Autodesk Inventor part; units mm, degrees
ref_plane "Work Plane1" through (-155.5267, -73.0733, 0) normal (-1, 0, 0) x (0, 0, 1)
ref_plane "YZ Plane" through (0, 0, 0) normal (1, 0, 0) x (0, 1, 0)
ref_plane "XZ Plane" through (0, 0, 0) normal (0, 1, 0) x (-1, 0, 0)
sketch "Sketch1" plane through (0, 0, 0) normal (0, 0, 1) x (1, 0, 0)
  line L0 (0, 0) -> (-28.5267, 28.5267) construction
  line L1 (-28.5267, 28.5267) -> (-79.3267, 28.5267)
  line L2 (-79.3267, -73.0733) -> (-28.5267, -123.8733)
  line L3 (-28.5267, -123.8733) -> (-28.5267, -149.2733)
  line L4 (-28.5267, -149.2733) -> (-104.7267, -73.0733)
  line L5 (-104.7267, -73.0733) -> (-104.7267, 79.3267)
  line L6 (-79.3267, -73.0733) -> (-79.3267, 28.5267)
  line L7 (-28.5267, 28.5267) -> (-28.5267, 79.3267)
  line L8 (-28.5267, 79.3267) -> (-104.7267, 79.3267)
  point P0 (-28.5267, 153.9136)
  dimension "d11" = 101.6
  dimension "d12" = 50.8
  dimension "d13" = 25.4
  dimension "d17" = 28.5267
  dimension "d18" = 50.8
  dimension "d23" = 135
  dimension "d24" = 17.9605
  dimension "d25" = 50.8
  dimension "d26" = 152.4
extrude "Extrusion1" add sketch "Sketch1" along normal blind 76.2
ref_plane "Work Plane1" through (-155.5267, -73.0733, 0) normal (-1, 0, 0) x (0, 0, 1)
sketch "Sketch2" plane through (-155.5267, -73.0733, 0) normal (-1, 0, 0) x (0, 0, 1)
  line L0 (0, -76.2) -> (76.2, -76.2)
  line L1 (76.2, -76.2) -> (50.8, -76.2)
  line L2 (76.2, 0) -> (76.2, 101.6)
  line L3 (50.8, -76.2) -> (76.2, 0)
  line L4 (76.2, 0) -> (76.2, -76.2)
  line L5 (0, 0) -> (0, -76.2)
  line L6 (0, -76.2) -> (25.4, -76.2)
  line L7 (25.4, -76.2) -> (0, 0)
  line L8 (0, 0) -> (0, -76.2)
  point P0 (0, 73.0733)
  dimension "d28" = 25.4
  dimension "d29" = 25.4
extrude "Extrusion2" cut sketch "Sketch2" against normal blind 177.8
sketch "Sketch3" plane through (-104.7267, 79.3267, 0) normal (0, 1, 0) x (1, 0, 0)
  circle A0 centre (38.1, -38.1) radius 8.7376
  line L0 (76.2, 0) -> (0, 0)
  line L1 (76.2, 0) -> (76.2, -76.2)
  point P0 (104.7267, 0)
  dimension "d32" = 38.1
  dimension "d33" = 38.1
  dimension "d34" = 17.4752
extrude "Extrusion3" cut sketch "Sketch3" against normal blind 6.35
sketch "Sketch4" plane through (-28.5267, 28.5267, 0) normal (1, 0, 0) x (0, 0, -1)
  circle A0 centre (-38.1, 25.4) radius 6.35
  line L0 (0, 0) -> (0, 50.8)
  line L1 (0, 0) -> (-76.2, 0)
  point P0 (0, -28.5267)
  point P1 (-38.1, 0)
  dimension "d39" = 12.7
  dimension "d40" = 38.1
  dimension "d41" = 25.4
extrude "Extrusion4" cut sketch "Sketch4" against normal blind 153.9875
sketch "Sketch5" plane through (-66.6267, 72.9767, 38.1) normal (0, 1, 0) x (1, 0, 0)
  circle A0 centre (0, 0) radius 3.175
  point P0 (66.6267, 38.1)
  dimension "d44" = 6.35
extrude "Extrusion5" cut sketch "Sketch5" against normal blind 3.175
properties part number "Claw_Finger_BR" material "PET Plastic"
Check sheet for the modelled part. Datum: model origin and axes. Units: mm. A direction names the side the tool comes from. Coordinates: 2 decimals unless noted, no trailing zeros. Order: outer loops, then holes, each group sorted by start corner. A loop starts at its lowest first (then second) coordinate and runs counter-clockwise, first axis right, second up. Notation, with made-up numbers: M 28.25,-38 L 81.25,-38 A17 cw 81.25,-18 Z; hole C 3.5,77.5 d4. An arc over 180 degrees is marked long. One line per question, with ' | ' between items. Start each with the question number.
Item 1: Mould release check, pull along X, two halves, no side actions. Record for faces 1 (the flat face through (-54.3, -98.1, 37.6)), 2 (the flat face through (-67, 69.802, 38)), 3 (the cylindrical face through (-61.93, 76.2, 30.73)), 4 (the flat face through (-84, 21, 76.2)): pulls with the +X half, pulls with the -X half, needs draft (parallel to the pull), parting line crosses it, or undercut.
Item 2: Material ranges on line 1 (X direction, y = 71, z = 38); line 2 (Y direction, x = -60, z = 32.5); line 3 (X direction, y = 75, z = 38), recorded low to high.
Item 3: Sectioned sample at B-B on z = 38.1. Record the cut outline in (x, y), and give its area (3 significant figures).
Item 4: Sectioned sample at A-A on x = -46. Record the cut outline in (y, z).
Item 5: Access from +Z, -Z, +X, -X, +Y, -Y to the whole of each face (thin tool, end or side, straight path). Record for faces 5 (the flat face through (-104.727, 2, 38)), 6 (the flat face through (-54, 28.527, 38)), 7 (the cylindrical face through (-68.967, 71.411, 35.954)).
Item 6: Sectioned sample at C-C on x = -81.5. Record the cut outline in (y, z).
Item 7: Gauge pin test, flat ends, axial feed: P1, Ø1.5, axis at x = -51.5, y = -105, coming from the +Z side; P2, Ø4, axis at y = -21, z = 55.5, coming from the +X side; P3, Ø4, axis at x = -64, y = -93.5, coming from the -Z side. Record the tip position at first contact, or that the pin passes through.
Item 8: Sectioned sample at D-D on z = 68.5. Record the cut outline in (x, y).
Answer below:
1) face 1: pulls with the +X half | face 2: undercut | face 3: undercut | face 4: needs draft
2) line 1: x = -104.73 to -69.8, -63.45 to -28.53 | line 2: y = -117.8 to -92.4, 28.53 to 50.93, 56.92 to 72.98 | line 3: x = -104.73 to -75.36, -57.89 to -28.53
3) outline: M -104.73,-73.07 L -28.53,-149.27 L -28.53,-123.87 L -79.33,-73.07 L -79.33,28.53 L -28.53,28.53 L -28.53,47.58 L -104.73,47.58 Z; M -104.73,60.28 L -28.53,60.28 L -28.53,79.33 L -57.89,79.33 L -57.89,72.98 L -63.45,72.98 L -63.45,69.8 L -69.8,69.8 L -69.8,72.98 L -75.36,72.98 L -75.36,79.33 L -104.73,79.33 Z | area: 6,970 mm^2
4) outline: M -131.8,19.58 L -106.4,11.11 L -106.4,65.09 L -131.8,56.62 Z; M 28.53,0 L 79.33,0 L 79.33,76.2 L 28.53,76.2 Z; hole C 53.93,38.1 d12.7
5) face 5: +Z, -Z, -X, +Y, -Y | face 6: +Z, -Z, +X | face 7: +Y
6) outline: M -96.3,7.74 L -73.07,0 L 79.33,0 L 79.33,76.2 L -73.07,76.2 L -96.3,68.46 Z; hole C 53.93,38.1 d12.7
7) P1: stops at z = 65.81 | P2: stops at x = -79.33 | P3: stops at z = 6.14
8) outline: M -104.73,-73.07 L -81.63,-96.17 L -56.23,-96.17 L -79.33,-73.07 L -79.33,28.53 L -28.53,28.53 L -28.53,79.33 L -104.73,79.33 Z
